Autodesk Inventor part; units mm, degrees
ref_plane "Arbeitsebene1" through (16, 0, -183) normal (0, 0, -1) x (-1, 0, 0)
ref_plane "Arbeitsebene2" through (0, 16, 0) normal (0, 1, 0) x (-1, 0, 0)
ref_plane "YZ Plane" through (0, 0, 0) normal (1, 0, 0) x (0, 1, 0)
sketch "Skizze1" plane through (0, 0, 0) normal (0, 1, 0) x (-1, 0, 0)
  line L0 (-16, 23) -> (16, 23)
  line L1 (16, 23) -> (16, -23)
  line L2 (16, -23) -> (-16, -23)
  line L3 (-16, -23) -> (-16, 23)
  line L4 (-16, 23) -> (16, -23) construction
  line L5 (16, 23) -> (-16, -23) construction
  point P0 (0, 0)
  dimension "d0" = 46
  dimension "d1" = 32
extrude "Extrusion1" add sketch "Skizze1" along normal blind 32
sketch "Skizze2" plane through (16, 0, -23) normal (0, 0, -1) x (-1, 0, 0)
  line L0 (0, 0) -> (0, 32)
  line L1 (0, 0) -> (32, 0)
  line L2 (32, 24) -> (0, 24)
  line L3 (0, 24) -> (0, 8)
  line L4 (0, 8) -> (32, 8)
  line L5 (32, 8) -> (32, 24)
  point P0 (16, 0)
  point P1 (0, 16)
  point P2 (16, 0)
  point P3 (16, 0)
  point P4 (0, 16)
  point P5 (16, 8)
  point P6 (16, 0)
  point P7 (0, 16)
  point P8 (0, 24)
  point P9 (0, 8)
  dimension "d51" = 16
extrude "Extrusion2" add sketch "Skizze2" along normal blind 160
sketch "Skizze4" plane through (16, 0, 23) normal (1, 0, 0) x (0, 0, -1)
  line L0 (0, 24) -> (40, 24)
  line L1 (40, 24) -> (40, 8)
  line L2 (40, 8) -> (0, 8)
  line L3 (0, 8) -> (0, 24)
  line L4 (0, 0) -> (0, 32)
  point P0 (23, 0)
  point P1 (0, 16)
  dimension "d14" = 16
  dimension "d15" = 40
extrude "Extrusion4" cut sketch "Skizze4" against normal up to surface (32 mm away)
fillet "Rundung2" radius 8 2 edges at (0, 24, -23) (0, 8, -23)
ref_plane "Arbeitsebene1" through (16, 0, -183) normal (0, 0, -1) x (-1, 0, 0)
mirror "Spiegeln1" about plane through (16, 0, -183) normal (0, 0, -1) of "Extrusion2", "Extrusion1", "Extrusion4"
fillet "Rundung4" radius 8 2 edges at (0, 24, -343) (0, 8, -343)
sketch "Skizze7" plane through (16, 32, 0) normal (1, 0, 0) x (0, -1, 0)
  line L0 (24, 17) -> (24, 17)
  line L1 (8, 17) -> (24, 17)
  line L2 (8, 31) -> (8, 335)
  point P0 (16, 183)
  point P1 (-9.4065, 183)
  point P2 (16, 17)
  point P3 (8, 183)
hole "Bohrung3" at (16, 16, -183) direction (-1, 0, 0) diameter 8 end through all
sketch "Skizze8" plane through (8, 8, -31) normal (0, -1, 0) x (0, 0, -1)
  line L0 (12, -8) -> (124, -8) construction
  line L1 (12, -16) -> (124, -16)
  line L2 (124, 0) -> (12, 0)
  arc A0 (12, 0) -> (12, -16) centre (12, -8) ccw
  arc A1 (124, -16) -> (124, 0) centre (124, -8) ccw
  line L3 (180, -8) -> (292, -8) construction
  line L4 (180, -16) -> (292, -16)
  line L5 (292, 0) -> (180, 0)
  arc A2 (180, 0) -> (180, -16) centre (180, -8) ccw
  arc A3 (292, -16) -> (292, 0) centre (292, -8) ccw
  line L6 (0, -24) -> (0, 8)
  line L7 (304, 8) -> (304, -24)
  line L8 (0, 8) -> (304, 8)
  point P0 (-31, 0)
  point P1 (68, -8)
  point P2 (236, -8)
  point P3 (0, -8)
  point P4 (304, -8)
  point P5 (152, -8)
  point P6 (152, 8)
  point P7 (0, -8)
  dimension "d43" = 112
  dimension "d46" = 112
  dimension "d47" = 16
  dimension "d48" = 16
  dimension "d55" = 28
  dimension "d56" = 28
extrude "Extrusion5" cut sketch "Skizze8" against normal up to surface (16 mm away)
sketch "Skizze9" plane through (0, 0, 0) normal (0, -1, 0) x (1, 0, 0)
  line L0 (-16, 23) -> (16, 23)
  arc A0 (8, -43) -> (-8, -43) centre (0, -43) ccw
  arc A1 (-8, -323) -> (8, -323) centre (0, -323) ccw
  point P0 (0, 0)
  point P1 (0, 7)
  point P2 (0, -373)
  point P3 (0, 23)
  dimension "d64" = 50
  dimension "d65" = 50
hole "Bohrung4" at (0, 0, 7) at (0, 0, -373) direction (0, 1, 0) diameter 12 depth 32
sketch "Skizze10" plane through (-16, 8, -31) normal (0, -1, 0) x (1, 0, 0)
  line L0 (32, 8) -> (0, 8)
  line L1 (32, 0) -> (32, -304)
  point P0 (16, 31)
  point P1 (16, -152)
  point P2 (16, 8)
  point P3 (32, -152)
hole "Bohrung5" at (0, 8, -183) direction (0, 1, 0) diameter 20 depth 16
sketch "Skizze11" plane through (-16, 0, -389) normal (0, -1, 0) x (1, 0, 0)
  circle A0 centre (16, 16) radius 6
  line L0 (0, 46) -> (0, 0)
  line L1 (32, 0) -> (32, 46)
  arc A1 (0, 16) -> (32, 16) centre (16, 16) ccw
  line L2 (32, 16) -> (0, 16)
  line L3 (0, 0) -> (32, 0)
  arc A2 (8, 66) -> (24, 66) centre (16, 66) ccw
  point P0 (16, 389)
  point P1 (16, 0)
  point P2 (16, 0)
  point P3 (16, 0)
  dimension "d73" = 16
  dimension "d74" = 50
extrude "Extrusion6" cut sketch "Skizze11" against normal up to surface (8 mm away) contours L1 L3 A1 | A1 L3 L0
ref_plane "Arbeitsebene2" through (0, 16, 0) normal (0, 1, 0) x (-1, 0, 0)
mirror "Spiegeln2" about plane through (0, 16, 0) normal (0, 1, 0) of "Extrusion6"
mirror "Spiegeln3" about plane through (16, 0, -183) normal (0, 0, -1) of "Extrusion6", "Spiegeln2"
equation "\"d48\" = d47"
properties part number "16" material "Kupfer, Legierung"
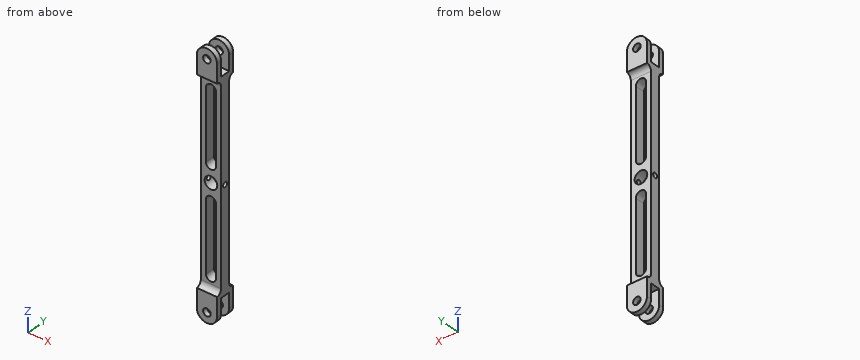
Geometry: final body of the model. Coordinates: model frame, mm. Coordinates: 2 decimals unless noted, no trailing zeros. Order: outer loops, then holes, each group sorted by start corner. A loop starts at its lowest first (then second) coordinate and runs counter-clockwise, first axis right, second up.
(1) First-contact query: pin 1 (16 mm diameter, centred on x = 0.5, z = -108.5, fed in from +Y); pin 2 (3 mm diameter, centred on x = -11, y = 22, fed in from -Z); pin 3 (1.5 mm diameter, centred on x = 3, y = 10.5, fed in from +Z). Flat tips, straight axial feed; report the tip coordinate or a pass-through.
(2) Section query C-C (x = 0). State how many separate pieces and enclosed holes the cut face has, plus the area to 3 significant figures.
(3) Section query A-A (z = -183). Return the cut outline in (x, y).
(4) Section query B-B (z = -289). Return the cut outline in (x, y).
(5) Material intervals for probe 1 along Y at (x, z) = (9.5, -358.5); probe 2 along X at (y, z) = (9.5, -296); probe 3 along Z at (x, y) = (2.5, 16.5), sorted ascending.
Solution:
1. pin 1: stops at y = 24
1. pin 2: stops at z = -349
1. pin 3: stops at z = -17
2. separate pieces: 8
2. enclosed holes: 0
2. area: 2,040 mm2
3. outline: (-16, 8) - (-10, 8) - (-10, 12) - (-16, 12) - close; (-16, 20) - (-10, 20) - (-10, 24) - (-16, 24) - close; (10, 8) - (16, 8) - (16, 12) - (10, 12) - close; (10, 20) - (16, 20) - (16, 24) - (10, 24) - close
4. outline: (-16, 8) - (-8, 8) - (-8, 24) - (-16, 24) - close; (8, 8) - (16, 8) - (16, 24) - (8, 24) - close
5. probe 1: y = 0 to 8, 24 to 32
5. probe 2: x = -16 to -8, 8 to 16
5. probe 3: z = -349 to -330.6, -203.4 to -192.68, -173.32 to -162.6, -35.4 to -17
